The drawing under review shows one solid part. Ordinate dimensions are in mm from its lowest x, y, z. A direction names the side the tool comes from. Coordinates: 2 decimals unless noted, no trailing zeros. Write each loop counter-clockwise with the first axis right and the second up, starting at its lowest first coordinate (ties: lowest second). Pieces come first, ordered by that corner, then holes.
Q1. Clearance check with a flat-ended pin moving along its axis: pin 1 Ø6 at (y, z) = (41.5, 40) entering from +X (1 decimal). State where the tip first meets the part, or that it passes through.
Q2. Add section A-A, the plane z = 39.5. Give the boundary of the cut face in (x, y), plus the area to 3 significant figures.
Q3. Add section C-C, the plane y = 32.5. Give the boundary of the cut face in (x, z), plus the area to 3 significant figures.
Q4. Add section B-B, the plane x = 85.5. Give the boundary of the cut face in (y, z), plus the area to 4 significant figures.
Q5. To check wall thickness, follow probe 1 along Y at (x, z) = (119.5, 25); probe 2 along Z at (x, y) = (28.5, 59); probe 3 along X at (y, z) = (14, 54) (1 decimal). State the ranges of each line that lie inside material, in increasing order.
Q6. Machinability: for the marked faces 1 and 2, which of the approach directions +Z, -Z, +X, -X, +Y, -Y give a long, thin tool a straight path to every point of the face, cutting with its end or side? Answer none if there is none.
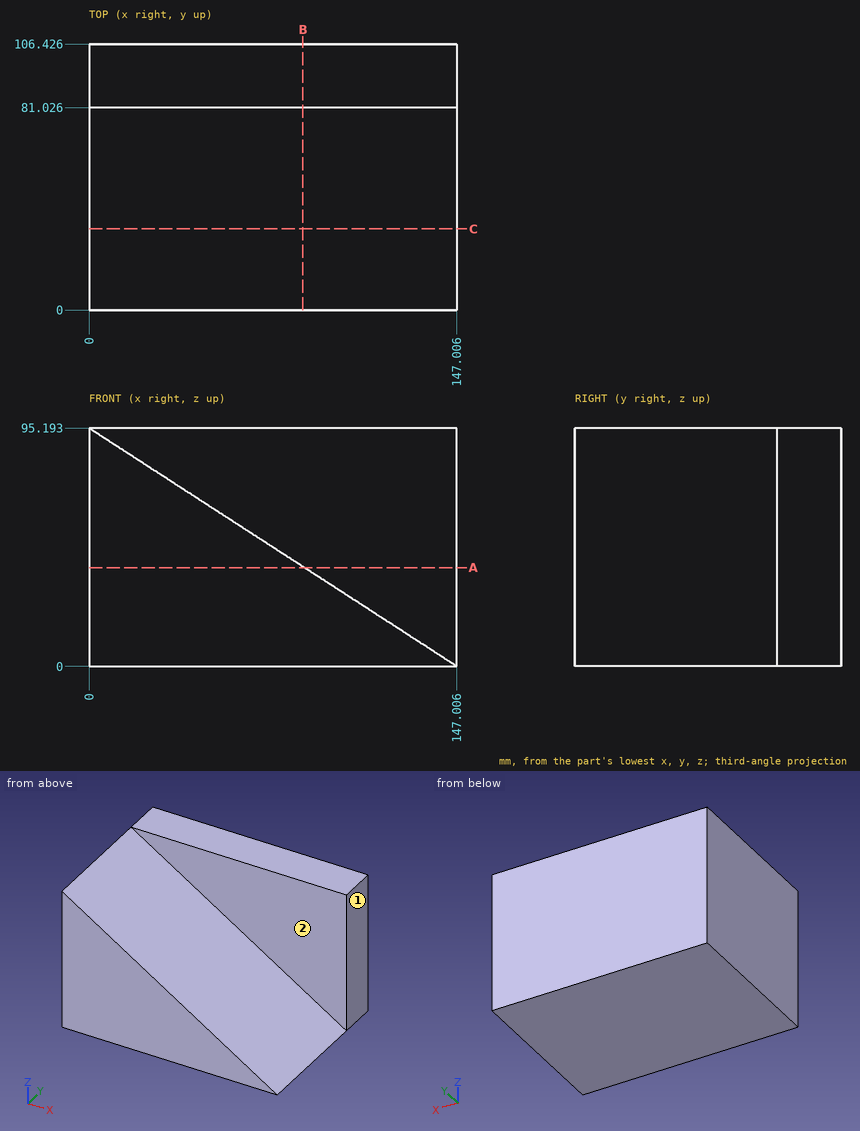
Here are the results:
1. pin 1: stops at x = 89.9
2. outline: (0, 0) - (86.01, 0) - (86.01, 81.03) - (147.01, 81.03) - (147.01, 106.43) - (0, 106.43) - close
2. area: 10,700 mm2
3. outline: (0, 0) - (147.01, 0) - (0, 95.19) - close
3. area: 7,000 mm2
4. outline: (0, 0) - (106.43, 0) - (106.43, 95.19) - (81.03, 95.19) - (81.03, 39.83) - (0, 39.83) - close
4. area: 5,645 mm2
5. probe 1: y = 81.03 to 106.43
5. probe 2: z = 0 to 76.74
5. probe 3: x = 0 to 63.6
6. face 1: +Z, -Z, +X, +Y, -Y
6. face 2: +Z, +X, -Y
